Read the model definition and answer for the solid it produces. Units are mm, in the model's axes. Face numbers are marked on the shaded views. Coordinates: 2 decimals unless noted, no trailing zeros. Loops run counter-clockwise (first coordinate to the right, second up) from the corner with the lowest first, then second, coordinate; pieces in that order, holes last. Notation, with made-up numbers: (88, 19.25) -> (92, 19.25) arc R26 ccw to (92, 34.25) -> close; hole circle Ø11 at (35, 54). An arc over 180 degrees is marked (long way). Answer as a JSON object with one key per item and string values. Group by question number.
Q1. The part is cut by section A-A on y = -11. Write down the section's boundary in (x, z), and give its area (3 significant figures).
Q2. The part is cut by section C-C on y = -1.5. Write down the section's boundary in (x, z), and give its area (3 significant figures).
Q3. Each of these flat-tipped pins is pushed along its axis until it touches: P1, Ø9, axis at x = 4, z = -1.5, coming from the -Y side; P2, Ø1, axis at y = -4, z = -27, coming from the +X side; P3, Ø2, axis at x = 18.75, z = 32.476, coming from the -Y side. Where does it stop, or does it pass through?
Q4. Straight lines are drawn through the part: line 1 along Z through (x, y) = (-18.75, -8.75); line 2 along Z through (x, y) = (0, -12.1); line 3 along Z through (x, y) = (-21, -7.5). For each, find the intervals that lie inside material, in ascending order. Write a range as [from, to].
Q5. Determine the mould class of the marked faces 1 and 2 for opening direction Z: released by +Z, released by -Z, zero draft, split by the parting line, or undercut.
Autodesk Inventor part; units mm, degrees
ref_plane "YZ Plane" through (0, 0, 0) normal (1, 0, 0) x (0, 1, 0)
ref_plane "XZ Plane" through (0, 0, 0) normal (0, 1, 0) x (-1, 0, 0)
ref_plane "XY Plane" through (0, 0, 0) normal (0, 0, 1) x (1, 0, 0)
sketch "Boceto1" plane through (0, 0, 0) normal (0, 1, 0) x (-1, 0, 0)
  circle A0 centre (0, 0) radius 50
  dimension "Diametro" = 100
extrude "Extrusión1" add sketch "Boceto1" against normal blind 8
fillet "Empalme1" radius 8 1 edges at (50, 0, 0)
sketch "Boceto2" plane through (0, -8, 0) normal (0, -1, 0) x (1, 0, 0)
  circle A0 centre (0, 0) radius 46
  circle A1 centre (0, 0) radius 50
  dimension "d22" = 4
extrude "Extrusión3" add sketch "Boceto2" along normal blind 6 contours A0
sketch "Boceto3" plane through (0, -14, 0) normal (0, -1, 0) x (1, 0, 0)
  circle A0 centre (0, 0) radius 9
  point P0 (-37.5, 0)
  point P1 (-18.75, -32.476)
  point P2 (18.75, -32.476)
  point P3 (37.5, 0)
  point P4 (18.75, 32.476)
  point P5 (-18.75, 32.476)
  dimension "d25" = 37.5
  dimension "d35" = 360
  dimension "d37" = 18
hole "Agujero2" at (-37.5, -14, 0) at (-18.75, -14, 32.476) at (-18.75, -14, -32.476) at (18.75, -14, 32.476) at (37.5, -14, 0) at (18.75, -14, -32.476) direction (0, 1, 0) diameter 2.459 depth 8.8
extrude "Extrusión4" cut sketch "Boceto3" against normal blind 5
properties part number "Tapa" material "Aluminio 6061"
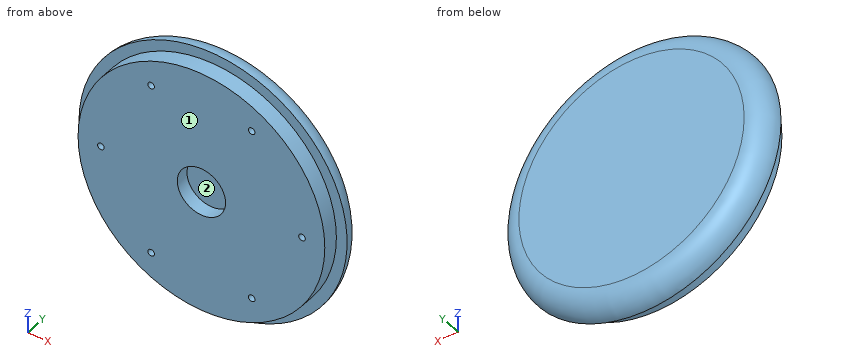
Final values:
{
 "1": {"outline": "circle Ø92 at (0, 0); hole circle Ø2.46 at (-37.5, 0); hole circle Ø2.46 at (-18.75, -32.48); hole circle Ø2.46 at (-18.75, 32.48); hole circle Ø18 at (0, 0); hole circle Ø2.46 at (18.75, -32.48); hole circle Ø2.46 at (18.75, 32.48); hole circle Ø2.46 at (37.5, 0)", "area": "6,360 mm2"},
 "2": {"outline": "circle Ø93.33 at (0, 0)", "area": "6,840 mm2"},
 "3": {"P1": "stops at y = -9", "P2": "stops at x = 41.27", "P3": "stops at y = -5.2"},
 "4": {"line 1": "z = [-42.01, -33.71], [-31.25, 31.25], [33.71, 42.01]", "line 2": "z = [-46, -9], [9, 46]", "line 3": "z = [-45.36, 45.36]"},
 "5": {"face 1": "zero draft", "face 2": "undercut"}
}
